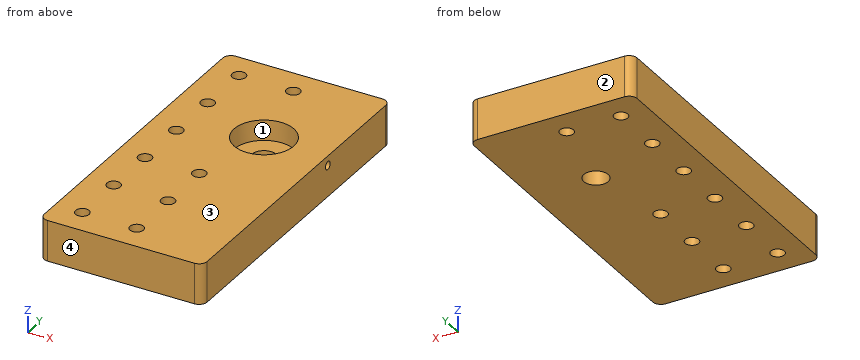
from build123d import *

# Parameters (mm, degrees)
SKETCH1_W               = 60
SKETCH1_H               = 120
SKETCH1_R               = 2.5
BOSS_EXTRUDE1_DEPTH     = 15
FILLET1_R               = 3
SKETCH2_R               = 4.5
CUT_EXTRUDE1_DEPTH      = 136
SKETCH2_3_R             = 11
SKETCH2_3_R_2           = 4.5
CUT_EXTRUDE2_DEPTH      = 7.5
CUT_EXTRUDE3_REACH      = 137
CUT_EXTRUDE3_END_RADIUS = 11
SKETCH3_R               = 1.5


with BuildPart() as part:
    # Sketch1 → Boss-Extrude1 (new body)
    with BuildSketch(Plane.XY):
        with Locations((30, 60)):
            Rectangle(SKETCH1_W, SKETCH1_H)
        with Locations((10, 110)):
            Circle(SKETCH1_R, mode=Mode.SUBTRACT)
        with Locations((30, 110)):
            Circle(SKETCH1_R, mode=Mode.SUBTRACT)
        with Locations((10, 90)):
            Circle(SKETCH1_R, mode=Mode.SUBTRACT)
        with Locations((10, 70)):
            Circle(SKETCH1_R, mode=Mode.SUBTRACT)
        with Locations((10, 10)):
            Circle(SKETCH1_R, mode=Mode.SUBTRACT)
        with Locations((30, 10)):
            Circle(SKETCH1_R, mode=Mode.SUBTRACT)
        with Locations((30, 50)):
            Circle(SKETCH1_R, mode=Mode.SUBTRACT)
        with Locations((10, 50)):
            Circle(SKETCH1_R, mode=Mode.SUBTRACT)
        with Locations((10, 30)):
            Circle(SKETCH1_R, mode=Mode.SUBTRACT)
        with Locations((30, 30)):
            Circle(SKETCH1_R, mode=Mode.SUBTRACT)
    extrude(amount=BOSS_EXTRUDE1_DEPTH)

    # Fillet1
    fillet1_edges = [part.edges().sort_by_distance(p)[0] for p in [
        (0, 120, 7.5),
        (60, 120, 7.5),
        (60, 0, 7.5),
        (0, 0, 7.5),
    ]]
    fillet(fillet1_edges, radius=FILLET1_R)

    # Sketch2 → Cut-Extrude1 (cut, through all)
    with BuildSketch(Plane.XY.offset(15)):
        with Locations((36.5, 80)):
            Circle(SKETCH2_R)
    extrude(amount=-CUT_EXTRUDE1_DEPTH, mode=Mode.SUBTRACT)

    # Sketch2<3> → Cut-Extrude2 (cut)
    with BuildSketch(Plane.XY.offset(15)):
        with Locations((36.5, 80)):
            Circle(SKETCH2_3_R)
        with Locations((36.5, 80)):
            Circle(SKETCH2_3_R_2, mode=Mode.SUBTRACT)
    extrude(amount=-CUT_EXTRUDE2_DEPTH, mode=Mode.SUBTRACT)

    # Cut-Extrude3: up to this cylinder (the profile starts outside it)
    cut_extrude3_end = Plane(origin=(36.5, 80, 11.5), z_dir=(0, 0, 1)) * Cylinder(CUT_EXTRUDE3_END_RADIUS, 297, mode=Mode.PRIVATE)
    # Sketch3 → Cut-Extrude3 (cut, up to the surface)
    with BuildSketch(Plane(origin=(60, 0, 0), x_dir=(0, 0, -1), z_dir=(1, 0, 0)), mode=Mode.PRIVATE) as cut_extrude3_sk1:
        with Locations((-11.5, 80)):
            Circle(SKETCH3_R)
    cut_extrude3_tool1 = extrude(cut_extrude3_sk1.sketch, amount=-CUT_EXTRUDE3_REACH, mode=Mode.PRIVATE) - cut_extrude3_end
    add(cut_extrude3_tool1.solids().sort_by_distance((60, 80, 11.5))[0], mode=Mode.SUBTRACT)


solid = part.part
Source: CAD feature listing. Evaluate the final solid. Frame: model axes, mm. Face numbers are marked on the shaded views. Round coordinates to 2 decimals unless told otherwise and drop trailing zeros. Loops run counter-clockwise (first coordinate to the right, second up) from the corner with the lowest first, then second, coordinate; pieces in that order, holes last.
Q1. Section C-C, the plane z = 3.5. State how many separate pieces and enclosed holes the cut face has, plus the area to 3 significant figures.
Q2. First-contact query: P1, Ø6.5, axis at x = 30, y = 10, coming from the -Z side. Flat tip, straight axial feed; report the tip coordinate or a pass-through.
Q3. Section A-A, the plane x = 10. Return loops of the section in (y, z), plus the area to 3 significant figures.
Q4. Mould query, pull axis Y, two halves, no side actions, for the marked faces 1, 2, 3 and 4. Classes: pulls with the +Y half, pulls with the -Y half, needs draft (parallel to the pull), parting line crosses it, or undercut.
Q5. Ray query, line 1 (Y direction, x = 36.5, z = 4.75); line 2 (Y direction, x = 30, z = 3.75); line 3 (X direction, y = 9.5, z = 8.75). Return the intervals inside material, ascending.
Q6. Section D-D, the plane x = 34.5. Return loops of the section in (y, z).
Q7. Section B-B, the plane y = 110. Return loops of the section in (x, z), plus the area to 3 significant figures.
Solutions:
1. separate pieces: 1
1. enclosed holes: 11
1. area: 6,930 mm2
2. P1: stops at z = 0
3. outline: (0, 0) - (7.5, 0) - (7.5, 15) - (0, 15) - close; (12.5, 0) - (27.5, 0) - (27.5, 15) - (12.5, 15) - close; (32.5, 0) - (47.5, 0) - (47.5, 15) - (32.5, 15) - close; (52.5, 0) - (67.5, 0) - (67.5, 15) - (52.5, 15) - close; (72.5, 0) - (87.5, 0) - (87.5, 15) - (72.5, 15) - close; (92.5, 0) - (107.5, 0) - (107.5, 15) - (92.5, 15) - close; (112.5, 0) - (120, 0) - (120, 15) - (112.5, 15) - close
3. area: 1,350 mm2
4. face 1: undercut
4. face 2: pulls with the +Y half
4. face 3: needs draft
4. face 4: pulls with the -Y half
5. line 1: y = 0 to 75.5, 84.5 to 120
5. line 2: y = 0 to 7.5, 12.5 to 27.5, 32.5 to 47.5, 52.5 to 107.5, 112.5 to 120
5. line 3: x = 0 to 7.55, 12.45 to 27.55, 32.45 to 60
6. outline: (0, 0) - (75.97, 0) - (75.97, 7.5) - (69.18, 7.5) - (69.18, 15) - (0, 15) - close; (84.03, 0) - (120, 0) - (120, 15) - (90.82, 15) - (90.82, 7.5) - (84.03, 7.5) - close
7. outline: (0, 0) - (7.5, 0) - (7.5, 15) - (0, 15) - close; (12.5, 0) - (27.5, 0) - (27.5, 15) - (12.5, 15) - close; (32.5, 0) - (60, 0) - (60, 15) - (32.5, 15) - close
7. area: 750 mm2
